Autodesk Inventor part; units mm, degrees
ref_plane "YZ Plane" through (0, 0, 0) normal (1, 0, 0) x (0, 1, 0)
ref_plane "XZ Plane" through (0, 0, 0) normal (0, 1, 0) x (-1, 0, 0)
ref_plane "XY Plane" through (0, 0, 0) normal (0, 0, 1) x (1, 0, 0)
sketch "Sketch1" plane through (0, 0, 0) normal (1, 0, 0) x (0, 1, 0)
  line L0 (0, 0) -> (24, 0)
  line L1 (24, 0) -> (24, -25)
  line L2 (24, -25) -> (0, -25)
  line L3 (0, -25) -> (0, 0)
  dimension "d0" = 24
  dimension "d1" = 25
extrude "Front Plate" add sketch "Sketch1" along normal blind 3
sketch "Sketch2" plane through (3, 0, 0) normal (1, 0, 0) x (0, 0, -1)
  line L0 (0, 24) -> (0, 0)
  line L1 (0, 21) -> (-3, 21)
  line L2 (-3, 21) -> (-3, 15)
  line L3 (-3, 15) -> (0, 15)
  line L4 (0, 15) -> (0, 21)
  line L5 (25, 24) -> (0, 24)
  line L6 (12.5, -1.4018) -> (12.5, 28.9484)
  line L7 (29.0475, 12) -> (-9.9529, 12)
  line L8 (0, 3) -> (-3, 3)
  line L9 (-3, 3) -> (-3, 9)
  line L10 (-3, 9) -> (0, 9)
  line L11 (0, 9) -> (0, 3)
  line L12 (0, 0) -> (25, 0)
  line L13 (3, 0) -> (9, 0)
  line L14 (9, 0) -> (9, -3)
  line L15 (9, -3) -> (3, -3)
  line L16 (3, -3) -> (3, 0)
  line L17 (25, 21) -> (28, 21)
  line L18 (28, 21) -> (28, 15)
  line L19 (28, 15) -> (25, 15)
  line L20 (25, 15) -> (25, 21)
  line L21 (25, 3) -> (28, 3)
  line L22 (28, 3) -> (28, 9)
  line L23 (28, 9) -> (25, 9)
  line L24 (25, 9) -> (25, 3)
  line L25 (22, 0) -> (16, 0)
  line L26 (16, 0) -> (16, -3)
  line L27 (16, -3) -> (22, -3)
  line L28 (22, -3) -> (22, 0)
  point P0 (0, 9)
  point P1 (9, 0)
  point P2 (0, 15)
  dimension "d4" = 3
  dimension "d5" = 6
  dimension "d6" = 3
  dimension "d7" = 3
  dimension "d8" = 6
  dimension "d9" = 3
extrude "Pegs" add sketch "Sketch2" against normal blind 3 contours L12 L28 L27 L26 | L0 L3 L2 L1 | L0 L8 L9 L10 | L14 L15 L16 L12 | L17 L18 L19 L20 | L24 L23 L22 L21
sketch "Sketch3" plane through (3, 0, 0) normal (1, 0, 0) x (0, 0, -1)
  line L0 (6, 19.2) -> (19, 19.2)
  line L1 (19, 19.2) -> (19, 2)
  line L2 (19, 2) -> (6, 2)
  line L3 (6, 2) -> (6, 19.2)
  line L4 (25, 9) -> (25, 15)
  line L5 (0, 15) -> (0, 9)
  line L6 (25, 24) -> (0, 24)
  line L7 (9, 0) -> (16, 0)
  point P0 (0, 0)
  dimension "d12" = 6
  dimension "d13" = 6
  dimension "d14" = 4.8
  dimension "d15" = 2
extrude "Camera CutOut" cut sketch "Sketch3" against normal blind 3
fillet "PiCam Corner Radius" radius 2 4 edges at (1.5, 24, 0) (1.5, 24, -25) (1.5, 0, -25) (1.5, 0, 0)
fillet "Peg Fillet" radius 1 12 edges at (1.5, 21, 3) (1.5, 15, 3) (1.5, 9, 3) (1.5, 3, 3) (1.5, -3, -3) (1.5, -3, -9) (1.5, -3, -16) (1.5, -3, -22) (1.5, 3, -28) (1.5, 9, -28) (1.5, 15, -28) (1.5, 21, -28)
equation "\"d0\" = CameraHeight"
equation "\"d1\" = CameraWidth"
equation "\"d2\" = Acrylic"
equation "\"d4\" = Acrylic"
equation "\"d5\" = 0.25 * CameraHeight"
equation "\"d7\" = Acrylic"
equation "\"d8\" = d5"
equation "\"d9\" = d6"
equation "\"d10\" = Acrylic"
equation "\"d13\" = d12"
equation "\"d16\" = Acrylic"
properties part number "FacePlate"
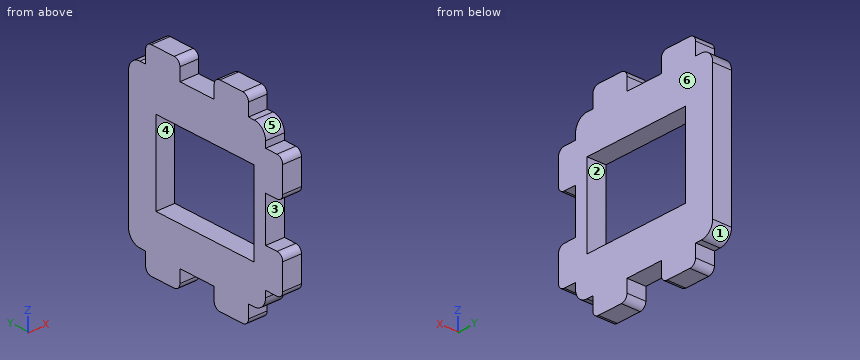
Design review of the part built by this model. Coordinates are the model's own, in mm. Face numbers are marked on the shaded views. A direction names the side the tool comes from. Coordinates: 2 decimals unless noted, no trailing zeros. Order: outer loops, then holes, each group sorted by start corner. A loop starts at its lowest first (then second) coordinate and runs counter-clockwise, first axis right, second up.
Item 1: Take a section at A-A, the plane z = -17.5. Write out the cut boundary in (x, y), then the cut area to 3 significant figures.
Item 2: The part is to be moulded in two halves that separate along Y. For the marked faces 4, 5 and 6, say which applies: pulls with the +Y half, pulls with the -Y half, needs draft (parallel to the pull), parting line crosses it, or undercut.
Item 3: For the marked faces 1, 2 and 3, list the 3-axis set-ups (+Z, -Z, +X, -X, +Y, -Y) from which the entire face can be reached by the end or side of a thin tool; tool diameter is ignored.
Item 4: Take a section at D-D, the plane z = -22.5. Write out the cut boundary in (x, y), then the cut area to 3 significant figures.
Item 5: For pin 1 Ø1.5 at (x, y) = (2, 11) entering from +Z; pin 2 Ø1.5 at (x, z) = (1, -14.5) entering from -Y; pin 3 Ø0.6 at (x, y) = (2, -1) entering from +Z, all flat-tipped, find the tip position at first contact; note any pin that passes through.
Item 6: For line 1 (Z direction, x = 2.05, y = 14); line 2 (Y direction, x = 2.45, z = -13); line 3 (Z direction, x = 2.8, y = 18), list the stretches that pass through material, from the lowest coordinate up.
Item 7: Take a section at C-C, the plane y = 21.5. Write out the cut boundary in (x, z), then the cut area to 3 significant figures.
Item 8: Take a section at B-B, the plane y = 2.5. Write out the cut boundary in (x, z).
The answers:
1. outline: (0, -3) - (3, -3) - (3, 2) - (0, 2) - close; (0, 19.2) - (3, 19.2) - (3, 24) - (0, 24) - close
1. area: 29.4 mm2
2. face 4: undercut
2. face 5: pulls with the -Y half
2. face 6: needs draft
3. face 1: -Z, +X, -X, +Y
3. face 2: +X, -X
3. face 3: +X, -X, -Y
4. outline: (0, 0) - (3, 0) - (3, 24) - (0, 24) - close
4. area: 72.0 mm2
5. pin 1: stops at z = 0
5. pin 2: stops at y = 0
5. pin 3: stops at z = -3
6. line 1: z = -25 to -19, -6 to 0
6. line 2: y = 0 to 2, 19.2 to 24
6. line 3: z = -28 to -19, -6 to 3
7. outline: (0, -25) - (3, -25) - (3, 0) - (0, 0) - close
7. area: 75.0 mm2
8. outline: (0, -25) - (3, -25) - (3, -19) - (0, -19) - close; (0, -6) - (3, -6) - (3, 0) - (0, 0) - close
